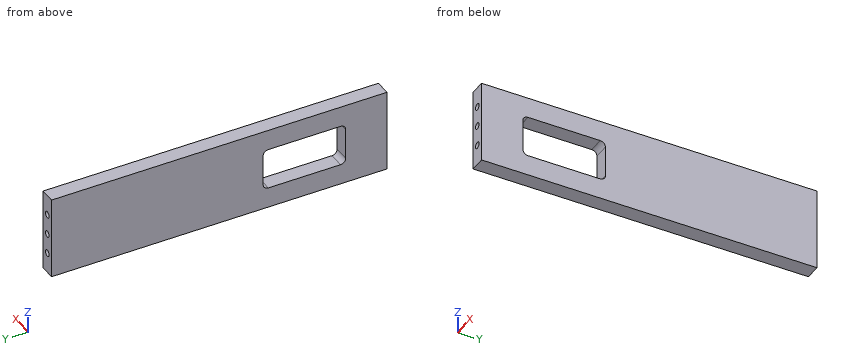
```python
from build123d import *

# Parameters (mm, degrees)
F0_W     = 206.375
F0_H     = 50.8
F0_W_2   = 50.8
F0_H_2   = 25.4
F1_DEPTH = 9.525
F3_D     = 3.96875
F3_DEPTH = 19.05
F3_TIP   = 1.1923327909
F5_D     = 3.96875
F5_DEPTH = 19.05
F5_TIP   = 1.1923327909
F6_R     = 3.175


with BuildPart() as f1:
    # F0 (on Right) → F1 (new body)
    with BuildSketch(Plane.YZ):
        with Locations((103.1875, 25.4)):
            Rectangle(F0_W, F0_H)
        with Locations((50.8, 25.4)):
            Rectangle(F0_W_2, F0_H_2, mode=Mode.SUBTRACT)
    extrude(amount=F1_DEPTH)

    # F3
    with Locations(Plane(origin=(0, 206.375, 0), x_dir=(-1, 0, 0), z_dir=(0, 1, 0))):
        with Locations((-4.7625, 38.1), (-4.7625, 25.4), (-4.7625, 12.7)):
            Hole(F3_D / 2, depth=F3_DEPTH)
            with Locations((0, 0, -(F3_DEPTH + F3_TIP / 2))):  # 118° drill point
                Cone(0, F3_D / 2, F3_TIP, mode=Mode.SUBTRACT)

    # F5
    with Locations(Plane.XZ):
        with Locations((4.7625, 38.1), (4.7625, 25.4), (4.7625, 12.7)):
            Hole(F5_D / 2, depth=F5_DEPTH)
            with Locations((0, 0, -(F5_DEPTH + F5_TIP / 2))):  # 118° drill point
                Cone(0, F5_D / 2, F5_TIP, mode=Mode.SUBTRACT)

    # F6
    f6_edges = [f1.edges().sort_by_distance(p)[0] for p in [
        (4.7625, 76.2, 38.1),
        (4.7625, 25.4, 38.1),
        (4.7625, 25.4, 12.7),
        (4.7625, 76.2, 12.7),
    ]]
    fillet(f6_edges, radius=F6_R)


solid = f1.part
```
Can you work these out from the model? Positions are in its coordinate system, mm. Give positions to 0.01 mm unless a question says otherwise; leave off trailing zeros. Order: outer loops, then holes, each group sorted by start corner. A loop starts at its lowest first (then second) coordinate and runs counter-clockwise, first axis right, second up. Notation, with made-up numbers: M -24.5,-0.5 L 27.5,-0.5 A23 ccw 27.5,32.5 Z; hole C -18,-20.5 d1. An arc over 180 degrees is marked long. Write item = value, one per line. Start each with the question number.
Q1. Suppose I cut it at A-A (z = 30.5). Write out the boundary of the cut face in (x, y) (3 decimals).
Q2. I need wall thicknesses on probe 1 along Y at (x, z) = (1.5, 20) (3 decimals); probe 2 along X at (y, z) = (192.5, 38.1) (3 decimals); probe 3 along Z at (x, y) = (1, 60). Which ranges of each line are inside material? Lowest first, please. Write a range as [from, to].
Q3. Will these pins go through, and if not, where does the flat tip stop? pin 1 Ø3.5 at (x, z) = (4.76, 38.1) entering from -Y; pin 2 Ø2.5 at (x, z) = (4.76, 25.4) entering from -Y; pin 3 Ø3.5 at (x, z) = (4.76, 25.4) entering from +Y.
Q4. Suppose I cut it at B-B (y = 51). Write out the boundary of the cut face in (x, z) (3 decimals), plus the area to 3 significant figures.
Check result:
q1.outline = M 0,0 L 9.525,0 L 9.525,25.4 L 0,25.4 Z; M 0,76.2 L 9.525,76.2 L 9.525,206.375 L 0,206.375 Z
q2.probe_1 = [0, 25.4], [76.2, 206.375]
q2.probe_2 = [0, 2.778], [6.747, 9.525]
q2.probe_3 = [0, 12.7], [38.1, 50.8]
q3.pin_1 = 19.19
q3.pin_2 = 19.49
q3.pin_3 = 187.19
q4.outline = M 0,0 L 9.525,0 L 9.525,12.7 L 0,12.7 Z; M 0,38.1 L 9.525,38.1 L 9.525,50.8 L 0,50.8 Z
q4.area = 242 mm2
